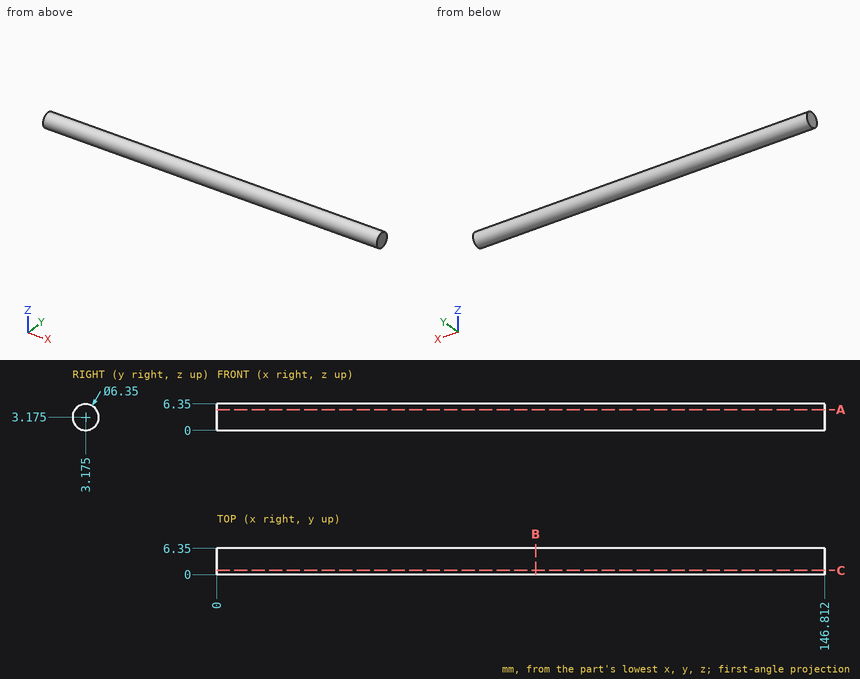
Check sheet for the drawn part. Datum: minimum x, y, z corner. Units: mm. Give positions to 0.01 mm unless a question says otherwise; leave off trailing zeros. Write each loop counter-clockwise with the first axis right and the second up, starting at its lowest first coordinate (ties: lowest second). Pieces come first, ordered by that corner, then holes.
(1) Cross-section at B-B (x = 77). Enter the section's corners in (y, z) (3 decimals).
(2) Gauge pin test, flat end, axial feed: pin 1 (2 mm diameter, centred on x = 37.5, z = 5, fed in from -Y). Record the tip position at first contact, or that the pin passes through.
(3) Cross-section at A-A (z = 5). Enter the section's corners in (x, y), plus the area to 3 significant figures.
(4) Material ranges on line 1 (Y direction, x = 78.5, z = 3.25); line 2 (Z direction, x = 10.5, y = 3.5); line 3 (Y direction, x = 88, z = 1.5), recorded low to high.
(5) Cross-section at C-C (y = 1). Enter the section's corners in (x, z).
Worked out:
1. outline: circle Ø6.35 at (3.175, 3.175)
2. pin 1: stops at y = 0.11
3. outline: (0, 0.58) - (146.81, 0.58) - (146.81, 5.77) - (0, 5.77) - close
3. area: 763 mm2
4. line 1: y = 0 to 6.35
4. line 2: z = 0.02 to 6.33
4. line 3: y = 0.48 to 5.87
5. outline: (0, 0.86) - (146.81, 0.86) - (146.81, 5.49) - (0, 5.49) - close
